Verification items for the finished model (mm, model axes). Give positions to 0.01 mm unless a question says otherwise; leave off trailing zeros. Loops run counter-clockwise (first coordinate to the right, second up) from the corner with the lowest first, then second, coordinate; pieces in that order, holes last. Notation, with made-up numbers: (60, 81.25) - (83, 81.25) arc R25 cw to (83, 100.25) - close; hole circle Ø2 at (69.5, 31.25). An arc over 180 degrees is marked (long way). Use one line per item in the form item = value.
```python
from build123d import *

# Parameters (mm, degrees)
SK_TOP_W             = 60
SK_TOP_H             = 63
EX_TOP_DEPTH         = 23.5
SK_RAILBOLTS_R       = 2.15
CUT_RAILBOLTS_DEPTH  = 8
SK_INSERTS_M4_R      = 2.8
CUT_INSERTS_M4_DEPTH = 8.1


with BuildPart() as part:
    # SK_Top → EX_Top (new body)
    with BuildSketch(Plane(origin=(0, 0, 0), x_dir=(1, 0, 0), z_dir=(0, 1, 0))):
        with Locations((0, -6.5)):
            Rectangle(SK_TOP_W, SK_TOP_H)
    extrude(amount=EX_TOP_DEPTH)

    # SK_RailBolts → CUT_RailBolts (cut)
    with BuildSketch(Plane.XY.offset(38)):
        with Locations((15, 13.5)):
            Circle(SK_RAILBOLTS_R)
        with Locations((-15, 13.5)):
            Circle(SK_RAILBOLTS_R)
    extrude(amount=-CUT_RAILBOLTS_DEPTH, mode=Mode.SUBTRACT)

    # SK_Inserts_M4 → CUT_Inserts_M4 (cut)
    with BuildSketch(Plane(origin=(0, 0, 0), x_dir=(1, 0, 0), z_dir=(0, 1, 0))):
        with Locations(Location((15, -15, 0), (0, 0, 270))):
            Circle(SK_INSERTS_M4_R)
        with Locations(Location((-15, -15, 0), (0, 0, 270))):
            Circle(SK_INSERTS_M4_R)
        with Locations(Location((15, 15, 0), (0, 0, 270))):
            Circle(SK_INSERTS_M4_R)
        with Locations(Location((-15, 15, 0), (0, 0, 270))):
            Circle(SK_INSERTS_M4_R)
    extrude(amount=CUT_INSERTS_M4_DEPTH, mode=Mode.SUBTRACT)


solid = part.part
```
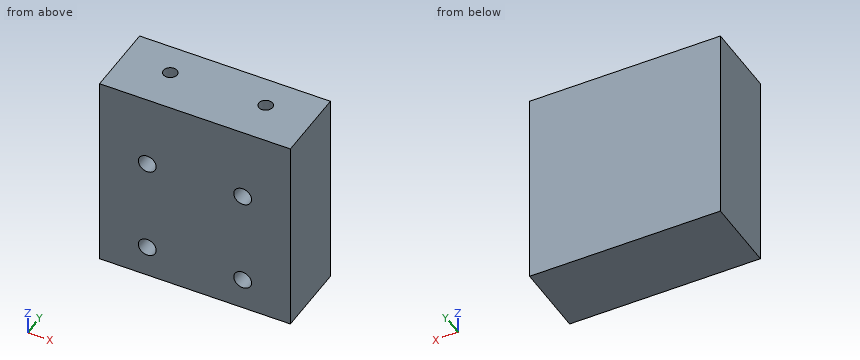
1. Depth check by flat-ended pin: pin 1 Ø3.5 at (x, y) = (15, 13.5) entering from +Z; pin 2 Ø1.7 at (x, z) = (-14.5, -15.5) entering from -Y. Enter the tip coordinate at first touch or a pass-through.
Result set:
pin_1 = 30
pin_2 = 8.1
2. Scan lines: probe 1 along X at (y, z) = (5, 15); probe 2 along Z at (x, y) = (-17.5, 6.75); probe 3 along Y at (x, z) = (-15, 35.5). Record each from-to range of solid material in increasing order.
Result set:
probe_1 = -30 to -17.8, -12.2 to 12.2, 17.8 to 30
probe_2 = -25 to -16.26, -13.74 to 13.74, 16.26 to 38
probe_3 = 0 to 11.35, 15.65 to 23.5
3. Section check D-D, the plane y = 13.5. Record the cut outline in (x, z), then the cut area to 3 significant figures.
Result set:
outline = (-30, -25) - (30, -25) - (30, 38) - (17.15, 38) - (17.15, 30) - (12.85, 30) - (12.85, 38) - (-12.85, 38) - (-12.85, 30) - (-17.15, 30) - (-17.15, 38) - (-30, 38) - close
area = 3,710 mm²
4. Section check C-C, the plane x = -15. Record the cut outline in (y, z).
Result set:
outline = (0, -25) - (23.5, -25) - (23.5, 38) - (15.65, 38) - (15.65, 30) - (11.35, 30) - (11.35, 38) - (0, 38) - (0, 17.8) - (8.1, 17.8) - (8.1, 12.2) - (0, 12.2) - (0, -12.2) - (8.1, -12.2) - (8.1, -17.8) - (0, -17.8) - close
5. Section check A-A, the plane y = 3. Record the cut outline in (x, z).
Result set:
outline = (-30, -25) - (30, -25) - (30, 38) - (-30, 38) - close; hole circle Ø5.6 at (-15, -15); hole circle Ø5.6 at (-15, 15); hole circle Ø5.6 at (15, -15); hole circle Ø5.6 at (15, 15)
6. Section check B-B, the plane z = -15. Record the cut outline in (x, y).
Result set:
outline = (-30, 0) - (-17.8, 0) - (-17.8, 8.1) - (-12.2, 8.1) - (-12.2, 0) - (12.2, 0) - (12.2, 8.1) - (17.8, 8.1) - (17.8, 0) - (30, 0) - (30, 23.5) - (-30, 23.5) - close
